Geometry check sheet. Reference: the model listing, model coordinates, mm. Face numbers are marked on the shaded views. A direction names the side the tool comes from. Round coordinates to 2 decimals unless told otherwise and drop trailing zeros. Loops run counter-clockwise (first coordinate to the right, second up) from the corner with the lowest first, then second, coordinate; pieces in that order, holes last. Notation, with made-up numbers: (-15, 8.5) - (4, 8.5) arc R6 cw to (4, 18.5) - close; hole circle Ø7 at (69, 60). An arc over 180 degrees is marked (long way). Answer as CSV lines item,"result". Start each with the question number.
1) Cross-section at B-B on y = 0. Record the boundary of the cut face in (x, z), and give its area (3 significant figures).
2) Cross-section at A-A on x = 0. Record the boundary of the cut face in (y, z).
3) Access from +Z, -Z, +X, -X, +Y, -Y to the whole of each face (thin tool, end or side, straight path). Record for the marked faces 1, 2, 3 and 4.
4) Draft check along X on the marked faces 5, 6, 7 and 8. Enter one of: released by +X, released by -X, zero draft, split by the parting line, or undercut.
5) Thickness scan on line 1 along Y through (x, z) = (0, 7); line 2 along X through (y, z) = (-19, 6.75) (3 decimals); line 3 along X through (y, z) = (11.5, 7.5). Record the ranges inside material, lowest first.
6) Depth check by flat-ended pin: P1, Ø6.5, axis at x = 18, z = 4.5, coming from the -Y side; P2, Ø3, axis at y = 1, z = 3, coming from the +X side; P3, Ø1, axis at y = 8, z = 2.5, coming from the +X side. Enter the tip coordinate at first touch or a pass-through.
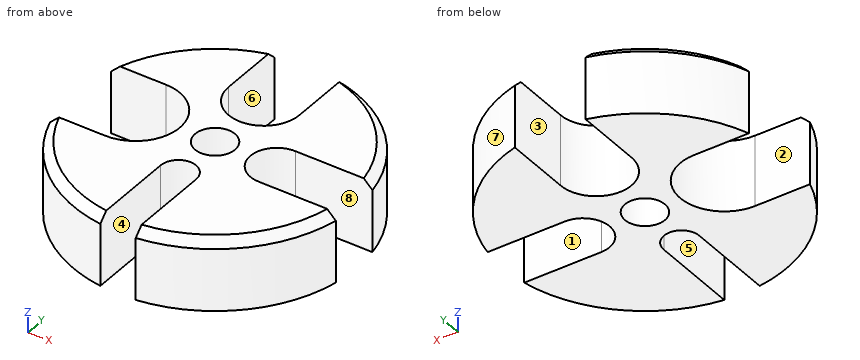
from build123d import *

# Parameters (mm, degrees)
F0_R     = 3.5814
F1_DEPTH = 12.7
F2_SIZE2 = 1.524
F2_SIZE  = 1.524


with BuildPart() as f1:
    # F0 (on Top) → F1 (new body)
    with BuildSketch(Plane.XY):
        with BuildLine():
            Line((-14.2748, -7.9375), (-24.127911, -7.9375))
            ThreePointArc((-24.127911, -7.9375), (-16.151392, -19.603381), (-3.175, -25.200781))
            Line((-3.175, -25.200781), (-3.175, -9.525))
            ThreePointArc((-3.175, -9.525), (0, -6.35), (3.175, -9.525))
            Line((3.175, -9.525), (3.175, -25.200781))
            ThreePointArc((3.175, -25.200781), (17.383268, -18.519773), (24.949521, -4.7625))
            Line((24.949521, -4.7625), (11.0998, -4.7625))
            ThreePointArc((11.0998, -4.7625), (6.3373, 0), (11.0998, 4.7625))
            Line((11.0998, 4.7625), (24.949521, 4.7625))
            ThreePointArc((24.949521, 4.7625), (18.52651, 17.376087), (6.35, 24.593444))
            Line((6.35, 24.593444), (6.35, 12.7))
            ThreePointArc((6.35, 12.7), (0, 6.35), (-6.35, 12.7))
            Line((-6.35, 12.7), (-6.35, 24.593444))
            ThreePointArc((-6.35, 24.593444), (-17.366084, 18.535887), (-24.127911, 7.9375))
            Line((-24.127911, 7.9375), (-14.2748, 7.9375))
            ThreePointArc((-14.2748, 7.9375), (-6.3373, 0), (-14.2748, -7.9375))
        make_face()
        Circle(F0_R, mode=Mode.SUBTRACT)
    extrude(amount=F1_DEPTH)

    # F2
    f2_edges = [f1.edges().sort_by_distance(p)[0] for p in [
        (-17.366084, 18.535887, 12.7),
        (18.52651, 17.376087, 12.7),
        (17.383268, -18.519773, 12.7),
        (-16.151392, -19.603381, 12.7),
    ]]
    chamfer(f2_edges, length=F2_SIZE, length2=F2_SIZE2)


solid = f1.part
Answer block:
1,outline,"(-6.34, 0) - (-3.58, 0) - (-3.58, 12.7) - (-6.34, 12.7) - close; (3.58, 0) - (6.34, 0) - (6.34, 12.7) - (3.58, 12.7) - close"
1,area,"70.0 mm^2"
2,outline,"(-6.35, 0) - (-3.58, 0) - (-3.58, 12.7) - (-6.35, 12.7) - close; (3.58, 0) - (6.35, 0) - (6.35, 12.7) - (3.58, 12.7) - close"
3,face 1,"+Z, -Z, +X"
3,face 2,"+Z, -Z, -X"
3,face 3,"+Z, -Z, +Y"
3,face 4,"+Z, -Z, -Y"
4,face 5,"undercut"
4,face 6,"undercut"
4,face 7,"released by +X"
4,face 8,"zero draft"
5,line 1,"y = -6.35 to -3.58, 3.58 to 6.35"
5,line 2,"x = -16.857 to -3.175, 3.175 to 16.857"
5,line 3,"x = -22.65 to -6.24, 6.24 to 22.65"
6,P1,"stops at y = -20.68"
6,P2,"stops at x = 7.05"
6,P3,"stops at x = 24.27"
